Build history of the part. All positions in model axes, mm. A direction names the side the tool comes from. Round coordinates to 2 decimals unless told otherwise and drop trailing zeros. Order: outer loops, then holes, each group sorted by start corner. A loop starts at its lowest first (then second) coordinate and runs counter-clockwise, first axis right, second up. Notation, with made-up numbers: M 18.5,-23.75 L 55.5,-23.75 A19 cw 55.5,-4.75 Z; hole C -5.5,-40 d8. An arc over 180 degrees is marked long. Use CSV: the item, a comma, the result in double quotes.
from build123d import *

# Parameters (mm, degrees)
SKETCH2_R           = 1.6
BOSS_EXTRUDE1_DEPTH = 7
FILLET1_R           = 2
FILLET2_R           = 2


with BuildPart() as part:
    # Sketch2 → Boss-Extrude1 (new body)
    with BuildSketch(Plane(origin=(0, -35.748750458, 0), x_dir=(1, 0, 0), z_dir=(0, 1, 0))):
        Polygon((-41.703283355, -38.480035415), (-41.703283355, -48.480035415), (-32.703283355, -48.480035415), (-24.703283355, -25.380229921), (-33.703283355, -25.380229921), (-33.703283355, -38.480035415), (-40.703283355, -38.480035415), align=None)
        with Locations(Location((-37.203283355, -43.480035415, 0), (0, 0, 270))):
            Circle(SKETCH2_R, mode=Mode.SUBTRACT)
        with Locations(Location((-29.203283355, -28.480035415, 0), (0, 0, 270))):
            Circle(SKETCH2_R, mode=Mode.SUBTRACT)
    extrude(amount=BOSS_EXTRUDE1_DEPTH)

    # Fillet1
    fillet1_edges = [part.edges().sort_by_distance(p)[0] for p in [
        (-24.703283355, -32.248750458, 25.380229921),
    ]]
    fillet(fillet1_edges, radius=FILLET1_R)

    # Fillet2
    fillet2_edges = [part.edges().sort_by_distance(p)[0] for p in [
        (-32.703283355, -32.248750458, 48.480035415),
        (-41.703283355, -32.248750458, 48.480035415),
        (-41.703283355, -32.248750458, 38.480035415),
        (-33.703283355, -32.248750458, 38.480035415),
    ]]
    fillet(fillet2_edges, radius=FILLET2_R)


solid = part.part
(1) Wall check: line 1 (X direction, y = -31.25, z = 29); line 2 (X direction, y = -30.5, z = 43.25); line 3 (Z direction, x = -37.5, y = -29.25). Give the ranges that are in metal, low to high. Write a range as from..to.
Answer block:
line 1,"x = -33.7..-30.72, -27.69..-25.96"
line 2,"x = -41.7..-38.79, -35.62..-30.89"
line 3,"z = 38.48..41.91, 45.05..48.48"
(2) Tool access for faces 1 (the face through (-28.976, -32.298, 37.718)), 2 (the face through (-38, -32, 38.48)): list every direction of +Z, -Z, +X, -X, +Y, -Y with a clear straight run to the whole face (end or side of a thin tool).
Answer block:
face 1,"+Z, +X, +Y, -Y"
face 2,"-Z, -X, +Y, -Y"
(3) Cut at A-A, the plane z = 28.75. Give the cut face in (x, y), and give its area (3 significant figures).
Answer block:
outline,"M -33.7,-35.75 L -30.78,-35.75 L -30.78,-28.75 L -33.7,-28.75 Z; M -27.63,-35.75 L -25.87,-35.75 L -25.87,-28.75 L -27.63,-28.75 Z"
area,"32.8 mm²"
(4) Drop flat-ended pins along their axis: pin 1 (2 mm diameter, centred on y = -33.5, z = 36, fed in from -X); pin 2 (2 mm diameter, centred on y = -31, z = 31.5, fed in from -X). Give the stop position or say it passes through.
Answer block:
pin 1,"stops at x = -33.77"
pin 2,"stops at x = -33.7"
(5) Two-plate mould, pull along Z, no slides. Class faces 3 (the face through (-31, -32, 25.38)), 4 (the face through (-36.7, -32.3, 45)), 5 (the face through (-41.703, -32, 43)): released by +Z, released by -Z, zero draft, split by the parting line, or undercut.
Answer block:
face 3,"released by -Z"
face 4,"undercut"
face 5,"zero draft"
(6) Cut at C-C, the plane x = -28.75. Give the cut face in (y, z).
Answer block:
outline,"M -35.75,25.38 L -28.75,25.38 L -28.75,26.95 L -35.75,26.95 Z; M -35.75,30.01 L -28.75,30.01 L -28.75,37.07 L -35.75,37.07 Z"
(7) Cut at D-D, the plane z = 34.75. Give the cut face in (x, y), and give its area (3 significant figures).
Answer block:
outline,"M -33.7,-35.75 L -27.95,-35.75 L -27.95,-28.75 L -33.7,-28.75 Z"
area,"40.3 mm²"
(8) Cut at B-B, the plane y = -31.5. Give the cut face in (x, z).
Answer block:
outline,"M -41.7,40.48 A2 ccw -39.7,38.48 L -35.7,38.48 A2 cw -33.7,36.48 L -33.7,25.38 L -27.51,25.38 A2 ccw -25.62,28.03 L -32.24,47.13 A2 ccw -34.13,48.48 L -39.7,48.48 A2 ccw -41.7,46.48 Z; hole C -37.2,43.48 d3.2; hole C -29.2,28.48 d3.2"
